```python
from build123d import *

# Parameters (mm, degrees)
BOSS_EXTRUDE1_DEPTH = 10
SKETCH3_R           = 14
BOSS_EXTRUDE2_DEPTH = 6
SKETCH4_R           = 2.75
SKETCH4_R_2         = 8
CUT_EXTRUDE1_DEPTH  = 16
FILLET1_R           = 1


with BuildPart() as part:
    # Sketch2 → Boss-Extrude1 (new body)
    with BuildSketch(Plane(origin=(0, 0, 0), x_dir=(0, 0, -1), z_dir=(1, 0, 0))):
        with BuildLine():
            Line((50, 7), (29.091106, 0.611092))
            ThreePointArc((29.091106, 0.611092), (25, 0), (20.908894, 0.611092))
            Line((20.908894, 0.611092), (0, 7))
            Line((0, 7), (0, 21))
            Line((0, 21), (20.908894, 27.388908))
            ThreePointArc((20.908894, 27.388908), (25, 28), (29.091106, 27.388908))
            Line((29.091106, 27.388908), (50, 21))
            Line((50, 21), (50, 7))
        make_face()
    extrude(amount=BOSS_EXTRUDE1_DEPTH)

    # Sketch3 → Boss-Extrude2 (add)
    with BuildSketch(Plane(origin=(10, 0, 0), x_dir=(0, 0, -1), z_dir=(1, 0, 0))):
        with Locations(Location((25, 14, 0), (0, 0, 253.008979))):
            Circle(SKETCH3_R)
    extrude(amount=BOSS_EXTRUDE2_DEPTH)

    # Sketch4 → Cut-Extrude1 (cut)
    with BuildSketch(Plane.ZY):
        with Locations((-45, 14)):
            Circle(SKETCH4_R)
        with Locations((-25, 14)):
            Circle(SKETCH4_R_2)
        with Locations((-5, 14)):
            Circle(SKETCH4_R)
    extrude(amount=-CUT_EXTRUDE1_DEPTH, mode=Mode.SUBTRACT)

    # Fillet1
    fillet1_edges = [part.edges().sort_by_distance(p)[0] for p in [
        (16, 27.388908, -29.091106),
        (16, 14, -33),
    ]]
    fillet(fillet1_edges, radius=FILLET1_R)


solid = part.part
```
Part model, mm, in its own coordinate system. Give positions to 0.01 mm unless a question says otherwise; leave off trailing zeros. Order: outer loops, then holes, each group sorted by start corner. A loop starts at its lowest first (then second) coordinate and runs counter-clockwise, first axis right, second up. Notation, with made-up numbers: M 2.5,43.25 L 45.5,43.25 A31 ccw 45.5,79.25 Z; hole C 87,-38 d6. An arc over 180 degrees is marked long. Use a Markdown table: item, result. Add a question column.
(1) Probe line 1 along X through (y, z) = (21, -42); line 2 along Y through (x, z) = (7.75, -5); line 3 along Y through (x, z) = (8.75, -25). List the from-to ranges inside material, lowest first. Write a range as [from, to].
(2) Saw through at C-C, the plane x = 3.75. Give the cut face in (y, z), and give its area (3 significant figures).
(3) Saw through at B-B, the plane y = 14. Give the cut face in (x, z).
(4) Mould opens along Z. For faces 1 (the face through (4.93, 3.76, -10.6)), 2 (the face through (4.93, 16.727, -5.358)), 3 (the face through (4.93, 24.24, -39.4)), 4 (the face through (7, 14, -33)) say: +Z half, -Z half, draft (parallel to the pull), parting line (faces both ways), or undercut.
(5) Saw through at A-A, the plane z = -25. Give the cut face in (x, y), and give its area (3 significant figures).
(6) Drop flat-ended pins along their axis: P1, Ø3, axis at x = 4.5, z = -6, coming from the -Y side; P2, Ø5, axis at x = 13.5, y = 12.5, coming from the +Z side; P3, Ø1, axis at x = 13.5, y = 16, coming from the +Z side; P4, Ø3.5, axis at y = 14, z = -5, coming from the +X side (1 decimal). Give the stop position or say it passes through.
(7) Saw through at D-D, the plane z = -45. Give the cut face in (x, y).
Answer key:
| question | item | result |
|---|---|---|
| 1 | line 1 | [0, 10] |
| 1 | line 2 | [5.47, 11.25], [16.75, 22.53] |
| 1 | line 3 | [0, 6], [22, 28] |
| 2 | outline | M 0.61,-29.09 L 7,-50 L 21,-50 L 27.39,-29.09 A14 ccw 27.39,-20.91 L 21,0 L 7,0 L 0.61,-20.91 A14 ccw Z; hole C 14,-25 d16; hole C 14,-45 d5.5; hole C 14,-5 d5.5 |
| 2 | area | 830 mm^2 |
| 3 | outline | M 0,-50 L 10,-50 L 10,-47.75 L 0,-47.75 Z; M 0,-42.25 L 10,-42.25 L 10,-39 L 15,-39 A1 ccw 16,-38 L 16,-34 A1 ccw 15,-33 L 0,-33 Z; M 0,-17 L 15,-17 A1 ccw 16,-16 L 16,-12 A1 ccw 15,-11 L 10,-11 L 10,-7.75 L 0,-7.75 Z; M 0,-2.25 L 10,-2.25 L 10,0 L 0,0 Z |
| 4 | face 1 | +Z half |
| 4 | face 2 | undercut |
| 4 | face 3 | -Z half |
| 4 | face 4 | undercut |
| 5 | outline | M 0,0 L 15,0 A1 ccw 16,1 L 16,5 A1 ccw 15,6 L 0,6 Z; M 0,22 L 15,22 A1 ccw 16,23 L 16,27 A1 ccw 15,28 L 0,28 Z |
| 5 | area | 191 mm^2 |
| 6 | P1 | y = 4.71 |
| 6 | P2 | z = -11 |
| 6 | P3 | z = -11.08 |
| 6 | P4 | through |
| 7 | outline | M 0,5.47 L 10,5.47 L 10,11.25 L 0,11.25 Z; M 0,16.75 L 10,16.75 L 10,22.53 L 0,22.53 Z |
